Source: CAD feature listing. Evaluate the final solid. Frame: model axes, mm. Give positions to 0.01 mm unless a question says otherwise; leave off trailing zeros. Loops run counter-clockwise (first coordinate to the right, second up) from the corner with the lowest first, then second, coordinate; pieces in that order, holes last. Notation, with made-up numbers: (-17, 88) -> (-11, 88) arc R24 cw to (-11, 121) -> close; hole circle Ø8 at (65.25, 28). An arc over 180 degrees is marked (long way). Return JSON: item names as keys, results as strings. Group by question number.
(1) Ray query, line 1 (X direction, y = -0.5, z = 5.5); line 2 (Z direction, x = 27, y = 16.5). Return the intervals inside material, ascending. Write a range as from..to.
(2) Cut plane C-C on z = 3.25. Return loops of the section in (x, y), then the cut area to 3 significant figures.
(3) Cut plane B-B on z = 12.75. Return loops of the section in (x, y), then the cut area to 3 significant figures.
(4) Pin query (flat end, axial travel): pin 1 (1.5 mm diameter, centred on y = -7, z = 4.5, fed in from -X); pin 2 (2 mm diameter, centred on x = 22.5, z = 2.5, fed in from +Y); pin 3 (4 mm diameter, centred on y = 15.5, z = 5, fed in from -X). Return the tip coordinate at first contact, or that it passes through.
(5) Draft query along X for faces 1 (the face through (15, -15, 5)), 2 (the face through (19.998, 31.367, 6.779)), 3 (the face through (18.28, 28.67, 9.31)), 4 (the face through (26.5, -23.8, 15)). Return one class per face: released by +X, released by -X, zero draft, split by the parting line, or undercut.
```python
from build123d import *

# Parameters (mm, degrees)
F0_R     = 34
F0_R_2   = 12.5
F1_DEPTH = 5
F0_R_3   = 37.2
F2_DEPTH = 15
F3_R     = 1.25
F4_R     = 4.99999


# Not quite as in the source:
# - a fillet or chamfer is up to 0.001 mm smaller than in the source, because OpenCascade refuses the exact size


with BuildPart() as f1:
    # F0 (on Top) → F1 (new body)
    with BuildSketch(Plane.XY):
        Circle(F0_R)
        with Locations((0, 0.3778987616)):
            Circle(F0_R_2, mode=Mode.SUBTRACT)
    extrude(amount=F1_DEPTH)

    # F0 (on Top) → F2 (join)
    with BuildSketch(Plane.XY):
        Circle(F0_R_3)
        Circle(F0_R, mode=Mode.SUBTRACT)
    extrude(amount=F2_DEPTH)

    # F3
    f3_edges = [f1.edges().sort_by_distance(p)[0] for p in [
        (-34, 0, 15),
        (-37.2, 0, 15),
    ]]
    fillet(f3_edges, radius=F3_R)

    # F4 (radius 5 in the source; OpenCascade refuses exactly that, so slightly less here)
    f4_edges = [f1.edges().sort_by_distance(p)[0] for p in [
        (-12.5, 0.377899, 5),
    ]]
    fillet(f4_edges, radius=F4_R)


solid = f1.part
```
Answers:
{
 "1": {"line 1": "-37.2..-34, 34..37.2", "line 2": "0..5"},
 "2": {"outline": "circle Ø74.4 at (0, 0); hole circle Ø27.4 at (0, 0.38)", "area": "3,760 mm²"},
 "3": {"outline": "circle Ø74.4 at (0, 0); hole circle Ø68 at (0, 0)", "area": "716 mm²"},
 "4": {"pin 1": "x = -36.67", "pin 2": "y = 30.36", "pin 3": "x = -34.66"},
 "5": {"face 1": "undercut", "face 2": "split by the parting line", "face 3": "undercut", "face 4": "zero draft"}
}
